```python
from build123d import *

# Parameters (mm, degrees)
F1_DEPTH  = 12.7
F2_R      = 5.55625
F3_DEPTH  = 4
F4_R      = 12.7
F5_DEPTH  = 12.701
F6_SIZE   = 3.81
F8_DEPTH  = 6.35
F9_R      = 2.407749
F10_DEPTH = 6.351


with BuildPart() as f1:
    # F0 (on Front) → F1 (new body)
    with BuildSketch(Plane.XZ):
        with BuildLine():
            Line((89.876923, -36.251613), (101.6, 0))
            ThreePointArc((101.6, 0), (0, 16.019351), (-101.6, 0))
            Line((-101.6, 0), (-89.876923, -36.251613))
            ThreePointArc((-89.876923, -36.251613), (0, -22.080649), (89.876923, -36.251613))
        make_face()
    extrude(amount=F1_DEPTH)

    # F2 (on face) → F3 (cut)
    with BuildSketch(Plane.XZ.offset(12.7)):
        with Locations((0, -3.030649)):
            Circle(F2_R)
        with Locations((19.041072, -3.613812)):
            Circle(F2_R)
        with Locations((38.01077, -5.361116)):
            Circle(F2_R)
        with Locations((-38.01077, -5.361116)):
            Circle(F2_R)
        with Locations((-19.041072, -3.613812)):
            Circle(F2_R)
    extrude(amount=-F3_DEPTH, mode=Mode.SUBTRACT)

    # F4 (on face) → F5 (cut, through all)
    with BuildSketch(Plane.XZ.offset(12.7)):
        with Locations((77.441715, -12.821887)):
            Circle(F4_R)
        with Locations((-77.441715, -12.821887)):
            Circle(F4_R)
    extrude(amount=-F5_DEPTH, mode=Mode.SUBTRACT)

    # F6
    f6_edges = [f1.edges().sort_by_distance(p)[0] for p in [
        (-95.738462, -12.7, -18.125807),
        (95.738462, -12.7, -18.125807),
    ]]
    chamfer(f6_edges, length=F6_SIZE)

    # F7 (on face) → F8 (cut)
    with BuildSketch(Plane.XZ.offset(12.7)):
        Polygon((-29.21, 0.382625), (-25.21, 2.692027), (-25.21, 7.310829), (-29.21, 9.62023), (-33.21, 7.310829), (-33.21, 2.692027), align=None)
    extrude(amount=-F8_DEPTH, mode=Mode.SUBTRACT)

    # F9 (on face) → F10 (cut, through all)
    with BuildSketch(Plane.XZ.offset(6.35)):
        with Locations((-29.21, 5.001428)):
            Circle(F9_R)
    extrude(amount=-F10_DEPTH, mode=Mode.SUBTRACT)


solid = f1.part
```
CAD build for the part. Positions are in the model's coordinates, mm. A direction names the side the tool comes from. Round coordinates to 2 decimals unless told otherwise and drop trailing zeros. Order: outer loops, then holes, each group sorted by start corner. A loop starts at its lowest first (then second) coordinate and runs counter-clockwise, first axis right, second up. Notation, with made-up numbers: (51.25, -17) - (63.25, -17) arc R36 ccw to (63.25, 18) - close; hole circle Ø6 at (78, -14.75). An arc over 180 degrees is marked (long way). Answer as CSV lines item,"result". Start each with the question number.
1. Pull direction X, two halves, no side cores. Call faces 1 (the face through (24.174, -10.728, -5.742)), 2 (the face through (64.754, -6.439, -12.263)), 3 (the face through (-95.82, -4.38, -17.87)), 4 (the face through (-1, -12.7, -9)): +X half, -X half, draft (parallel to the pull), parting line (faces both ways), or undercut.
2. Drill centre lines: L1, parallel to X at y = -4.5, z = -13; L2, parallel to X at y = -4.5, z = -18; L3, parallel to Z at x = 77.5, y = -3.75. Where is each one in solid material? Low to high. Write a range as [from, to].
3. Saw through at C-C, the plane x = 0. Write the cut outline in (y, z), and give its area (3 significant figures).
4. Saw through at B-B, the plane z = -17.5. Write the cut outline in (x, y).
5. Pin check, flat tips, straight feed: pin 1 (3 mm diameter, centred on x = -60.5, y = -2.5, fed in from -Z); pin 2 (14.5 mm diameter, centred on x = 38.01, z = -5.36, fed in from -Y); pin 3 (23 mm diameter, centred on x = -77.44, z = -12.82, fed in from -Y); pin 4 (5.5 mm diameter, centred on x = -0.5, z = -4.5, fed in from -Y). Stop position of each tip, or through.
6. Saw through at D-D, the plane z = -28. Write the cut outline in (x, y).
7. Tool access for faces 5 (the face through (-31.615, -3.219, 5.107)), 6 (the face through (19, -8.7, -4)): list every direction of +Z, -Z, +X, -X, +Y, -Y with a clear straight run to the whole face (end or side of a thin tool).
8. Saw through at A-A, the plane y = -1.75. Write the cut outline in (x, z).
Model answer:
1,face 1,"undercut"
1,face 2,"undercut"
1,face 3,"-X half"
1,face 4,"draft"
2,L1,"x = [-97.4, -90.14], [-64.74, 64.74], [90.14, 97.4]"
2,L2,"x = [-95.78, -89.04], [-65.85, 65.85], [89.04, 95.78]"
2,L3,"z = [-32.55, -25.52], [-0.12, 6.8]"
3,outline,"(-12.7, -22.08) - (0, -22.08) - (0, 16.02) - (-12.7, 16.02) - (-12.7, 2.53) - (-8.7, 2.53) - (-8.7, -8.59) - (-12.7, -8.59) - close"
3,area,"439 mm²"
4,outline,"(-95.94, -8.89) - (-91.94, -12.7) - (-89.25, -12.7) - (-89.25, 0) - (-95.94, 0) - close; (-65.63, -12.7) - (65.63, -12.7) - (65.63, 0) - (-65.63, 0) - close; (89.25, -12.7) - (91.94, -12.7) - (95.94, -8.89) - (95.94, 0) - (89.25, 0) - close"
5,pin 1,"stops at z = -28.74"
5,pin 2,"stops at y = -12.7"
5,pin 3,"passes through"
5,pin 4,"stops at y = -8.7"
6,outline,"(-92.55, -8.89) - (-88.54, -12.7) - (-58.51, -12.7) - (-58.51, 0) - (-92.55, 0) - close; (58.51, -12.7) - (88.54, -12.7) - (92.55, -8.89) - (92.55, 0) - (58.51, 0) - close"
7,face 5,"+Y, -Y"
7,face 6,"-Y"
8,outline,"(-101.6, 0) - (-89.88, -36.25) arc R292.1 cw to (89.88, -36.25) - (101.6, 0) arc R330.2 ccw to start; hole circle Ø25.4 at (-77.44, -12.82); hole circle Ø4.82 at (-29.21, 5); hole circle Ø25.4 at (77.44, -12.82)"
